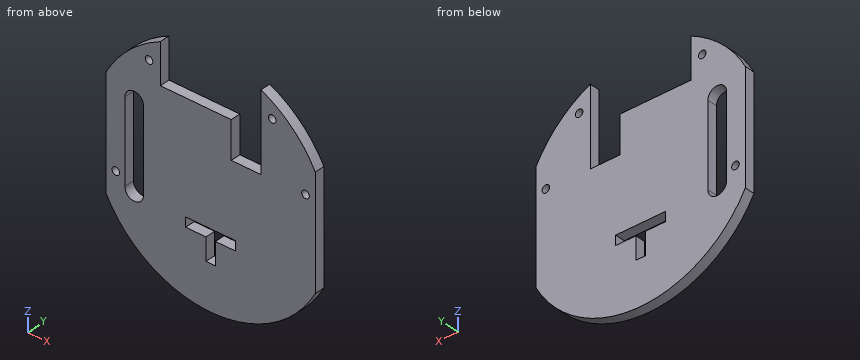
```python
from build123d import *

# Parameters (mm, degrees)
SKETCH1_W          = 13.4
SKETCH1_H          = 2.54
BASE_DEPTH         = 2.7
WHEEL_HOLE_REACH   = 44.441
SKETCH9_R          = 1.016
CHIP_HOLDING_DEPTH = 43.440952488
NUB_SLOT_REACH     = 44.441
SKETCH10_W         = 2.54
SKETCH10_H         = 6
SKETCH11_R         = 1
CUT_EXTRUDE1_DEPTH = 10


with BuildPart() as part:
    # Sketch1 → Base (new body)
    with BuildSketch(Plane(origin=(0, 0, 0), x_dir=(1, 0, 0), z_dir=(0, 1, 0))):
        with BuildLine():
            Line((28.033586073, 14.905722118), (28.033586073, -14.905722118))
            ThreePointArc((28.033586073, -14.905722118), (0, -31.75), (-28.033586073, -14.905722118))
            Line((-28.033586073, -14.905722118), (-28.033586073, 14.905722118))
            ThreePointArc((-28.033586073, 14.905722118), (0, 31.75), (28.033586073, 14.905722118))
        make_face()
        with Locations((0, 12.57)):
            Rectangle(SKETCH1_W, SKETCH1_H, mode=Mode.SUBTRACT)
    extrude(amount=BASE_DEPTH)

    # Sketch2 → Wheel Hole (cut, up to next)
    with BuildSketch(Plane(origin=(0, 2.7, 0), x_dir=(-1, 0, 0), z_dir=(0, 1, 0)), mode=Mode.PRIVATE) as wheel_hole_sk1:
        with BuildLine():
            Line((18, -11), (18, 11))
            ThreePointArc((18, 11), (20.5, 13.5), (23, 11))
            Line((23, 11), (23, -11))
            ThreePointArc((23, -11), (20.5, -13.5), (18, -11))
        make_face()
    wheel_hole_tool1 = extrude(wheel_hole_sk1.sketch, amount=-WHEEL_HOLE_REACH, mode=Mode.PRIVATE) & part.part
    add(wheel_hole_tool1.solids().sort_by_distance((-20.5, 2.7, 0))[0], mode=Mode.SUBTRACT)

    # Sketch9 → Chip Holding (cut, through all)
    with BuildSketch(Plane(origin=(0, 2.7, 0), x_dir=(-1, 0, 0), z_dir=(0, 1, 0))):
        with Locations(Location((25.4, -8.255, 0), (0, 0, 90))):
            Circle(SKETCH9_R)
        with Locations(Location((-25.4, 8.255, 0), (0, 0, 90))):
            Circle(SKETCH9_R)
    extrude(amount=-CHIP_HOLDING_DEPTH, mode=Mode.SUBTRACT)

    # Sketch10 → Nub Slot (cut, up to next)
    with BuildSketch(Plane.XZ, mode=Mode.PRIVATE) as nub_slot_sk1:
        with Locations((0, -16.84)):
            Rectangle(SKETCH10_W, SKETCH10_H)
    nub_slot_tool1 = extrude(nub_slot_sk1.sketch, amount=-NUB_SLOT_REACH, mode=Mode.PRIVATE) & part.part
    add(nub_slot_tool1.solids().sort_by_distance((0, 0, -16.84))[0], mode=Mode.SUBTRACT)

    # Sketch11 → Cut-Extrude1 (cut)
    with BuildSketch(Plane(origin=(0, 2.7, 0), x_dir=(1, 0, 0), z_dir=(0, 1, 0))):
        with Locations(Location((16.5, -22.91366528, 0), (0, 0, 270))):
            Circle(SKETCH11_R)
        with Locations(Location((-16.5, -22.91366528, 0), (0, 0, 270))):
            Circle(SKETCH11_R)
        Polygon((-13.5, -31.75), (13.5, -31.75), (13.5, -17.91366528), (13.5, -7.91366528), (5.5, -7.91366528), (5.5, -17.91366528), (-13.5, -17.91366528), align=None)
    extrude(amount=-CUT_EXTRUDE1_DEPTH, mode=Mode.SUBTRACT)


solid = part.part
```
Read the model definition and answer for the solid it produces. Units are mm, in the model's axes. Coordinates: 2 decimals unless noted, no trailing zeros. Write each loop counter-clockwise with the first axis right and the second up, starting at its lowest first coordinate (ties: lowest second). Pieces come first, ordered by that corner, then holes. Notation, with made-up numbers: (-40, 18) - (13, 18) arc R20 ccw to (13, 50) - close; hole circle Ø4 at (49, -8). An arc over 180 degrees is marked (long way). Answer as a JSON object with one key per item and string values. Group by question number.
1. A cutting plane is placed at A-A (z = -2.5). Determine the outline of the cut face in (x, y), plus the area to 3 significant figures.
2. Consider L1, parallel to X at y = 0.95, z = 11; L2, parallel to X at y = 0.3, z = -12.5; L3, parallel to X at y = 0.2, z = -3. Determine where each line is inside the solid, lowest interval first. Write a range as [from, to].
3. A cutting plane is placed at C-C (y = 0.6). Determine the outline of the cut face in (x, z) (3 decimals), plus the area to 3 significant figures.
4. A cutting plane is placed at B-B (x = -25.4). Determine the outline of the cut face in (y, z).
5. A cutting plane is placed at D-D (x = 10). Determine the outline of the cut face in (y, z), plus the area to 3 significant figures.
6. Each of these flat-tipped pins is pushed along its axis until it touches: P1, Ø0.8, axis at x = 1, y = 1.5, coming from the -Z side; P2, Ø0.8, axis at x = -4, y = 1.5, coming from the +Z side; P3, Ø1.4, axis at y = 1, z = 23, coming from the +X side. Where does it stop, or does it pass through?
Worked out:
{
 "1": {"outline": "(-28.03, 0) - (-23, 0) - (-23, 2.7) - (-28.03, 2.7) - close; (-18, 0) - (28.03, 0) - (28.03, 2.7) - (-18, 2.7) - close", "area": "138 mm²"},
 "2": {"L1": "x = [-28.03, -23], [-18, 5.5], [13.5, 28.03]", "L2": "x = [-28.03, -22.5], [-18.5, -6.7], [6.7, 28.03]", "L3": "x = [-28.03, -23], [-18, 28.03]"},
 "3": {"outline": "(-28.034, -14.906) arc R31.75 ccw to (28.034, -14.906) - (28.034, 14.906) arc R31.75 ccw to (13.5, 28.737) - (13.5, 7.914) - (5.5, 7.914) - (5.5, 17.914) - (-13.5, 17.914) - (-13.5, 28.737) arc R31.75 ccw to (-28.034, 14.906) - close; hole circle Ø2.032 at (-25.4, -8.255); hole (-23, -11) arc R2.5 ccw to (-18, -11) - (-18, 11) arc R2.5 ccw to (-23, 11) - close; hole circle Ø2 at (-16.5, 22.914); hole (-6.7, -13.84) - (-1.27, -13.84) - (-1.27, -19.84) - (1.27, -19.84) - (1.27, -13.84) - (6.7, -13.84) - (6.7, -11.3) - (-6.7, -11.3) - close; hole circle Ø2 at (16.5, 22.914); hole circle Ø2.032 at (25.4, 8.255)", "area": "2,400 mm²"},
 "4": {"outline": "(0, -19.05) - (2.7, -19.05) - (2.7, -9.27) - (0, -9.27) - close; (0, -7.24) - (2.7, -7.24) - (2.7, 19.05) - (0, 19.05) - close"},
 "5": {"outline": "(0, -30.13) - (2.7, -30.13) - (2.7, 7.91) - (0, 7.91) - close", "area": "103 mm²"},
 "6": {"P1": "stops at z = -31.74", "P2": "stops at z = 17.91", "P3": "stops at x = 22.6"}
}
